from build123d import *

# Parameters (mm, degrees)
SKETCH_2_R          = 1.6
EXTRUDE_1_DEPTH     = 3.8
CUT_EXTRUDE_1_REACH = 22.061
SKETCH_3_R          = 0.925
SKETCH_3_R_2        = 0.7
EXTRUDE_2_DEPTH     = 2


with BuildPart() as part:
    # Эскиз2 → Бобышка-Вытянуть1 (new body)
    with BuildSketch(Plane.XY):
        with BuildLine():
            Line((-14.886464029, 14), (-14.886464029, -14))
            ThreePointArc((-14.886464029, -14), (-10.886464029, -18), (-6.886464029, -14))
            Line((-6.886464029, -14), (-6.886464029, 14))
            ThreePointArc((-6.886464029, 14), (-10.886464029, 18), (-14.886464029, 14))
        make_face()
        with Locations(Location((-10.886464029, -14, 0), (0, 0, 180))):
            Circle(SKETCH_2_R, mode=Mode.SUBTRACT)
        with Locations(Location((-10.886464029, 14, 0), (0, 0, 180))):
            Circle(SKETCH_2_R, mode=Mode.SUBTRACT)
    extrude(amount=EXTRUDE_1_DEPTH)

    # Эскиз3 → Вырез-Вытянуть1 (cut, up to next)
    with BuildSketch(Plane.ZY.offset(14.886464029), mode=Mode.PRIVATE) as cut_extrude_1_sk1:
        with Locations((4, -10)):
            Circle(SKETCH_3_R)
    cut_extrude_1_tool1 = extrude(cut_extrude_1_sk1.sketch, amount=-CUT_EXTRUDE_1_REACH, mode=Mode.PRIVATE) & part.part
    # Эскиз3 → Вырез-Вытянуть1 (cut, up to next)
    with BuildSketch(Plane.ZY.offset(14.886464029), mode=Mode.PRIVATE) as cut_extrude_1_sk2:
        with Locations((4, -7.5)):
            Circle(SKETCH_3_R_2)
    cut_extrude_1_tool2 = extrude(cut_extrude_1_sk2.sketch, amount=-CUT_EXTRUDE_1_REACH, mode=Mode.PRIVATE) & part.part
    # Эскиз3 → Вырез-Вытянуть1 (cut, up to next)
    with BuildSketch(Plane.ZY.offset(14.886464029), mode=Mode.PRIVATE) as cut_extrude_1_sk3:
        with Locations((4, -5)):
            Circle(SKETCH_3_R_2)
    cut_extrude_1_tool3 = extrude(cut_extrude_1_sk3.sketch, amount=-CUT_EXTRUDE_1_REACH, mode=Mode.PRIVATE) & part.part
    # Эскиз3 → Вырез-Вытянуть1 (cut, up to next)
    with BuildSketch(Plane.ZY.offset(14.886464029), mode=Mode.PRIVATE) as cut_extrude_1_sk4:
        with Locations((4, 10)):
            Circle(SKETCH_3_R)
    cut_extrude_1_tool4 = extrude(cut_extrude_1_sk4.sketch, amount=-CUT_EXTRUDE_1_REACH, mode=Mode.PRIVATE) & part.part
    # Эскиз3 → Вырез-Вытянуть1 (cut, up to next)
    with BuildSketch(Plane.ZY.offset(14.886464029), mode=Mode.PRIVATE) as cut_extrude_1_sk5:
        with Locations((4, 7.5)):
            Circle(SKETCH_3_R_2)
    cut_extrude_1_tool5 = extrude(cut_extrude_1_sk5.sketch, amount=-CUT_EXTRUDE_1_REACH, mode=Mode.PRIVATE) & part.part
    # Эскиз3 → Вырез-Вытянуть1 (cut, up to next)
    with BuildSketch(Plane.ZY.offset(14.886464029), mode=Mode.PRIVATE) as cut_extrude_1_sk6:
        with Locations((4, 5)):
            Circle(SKETCH_3_R_2)
    cut_extrude_1_tool6 = extrude(cut_extrude_1_sk6.sketch, amount=-CUT_EXTRUDE_1_REACH, mode=Mode.PRIVATE) & part.part
    # Эскиз3 → Вырез-Вытянуть1 (cut, up to next)
    with BuildSketch(Plane.ZY.offset(14.886464029), mode=Mode.PRIVATE) as cut_extrude_1_sk7:
        with Locations((4, 2.5)):
            Circle(SKETCH_3_R)
    cut_extrude_1_tool7 = extrude(cut_extrude_1_sk7.sketch, amount=-CUT_EXTRUDE_1_REACH, mode=Mode.PRIVATE) & part.part
    # Эскиз3 → Вырез-Вытянуть1 (cut, up to next)
    with BuildSketch(Plane.ZY.offset(14.886464029), mode=Mode.PRIVATE) as cut_extrude_1_sk8:
        with Locations((4, 0)):
            Circle(SKETCH_3_R_2)
    cut_extrude_1_tool8 = extrude(cut_extrude_1_sk8.sketch, amount=-CUT_EXTRUDE_1_REACH, mode=Mode.PRIVATE) & part.part
    # Эскиз3 → Вырез-Вытянуть1 (cut, up to next)
    with BuildSketch(Plane.ZY.offset(14.886464029), mode=Mode.PRIVATE) as cut_extrude_1_sk9:
        with Locations((4, -2.5)):
            Circle(SKETCH_3_R)
    cut_extrude_1_tool9 = extrude(cut_extrude_1_sk9.sketch, amount=-CUT_EXTRUDE_1_REACH, mode=Mode.PRIVATE) & part.part
    add(cut_extrude_1_tool1.solids().sort_by_distance((-14.886464, -10, 4))[0], mode=Mode.SUBTRACT)
    add(cut_extrude_1_tool2.solids().sort_by_distance((-14.886464, -7.5, 4))[0], mode=Mode.SUBTRACT)
    add(cut_extrude_1_tool3.solids().sort_by_distance((-14.886464, -5, 4))[0], mode=Mode.SUBTRACT)
    add(cut_extrude_1_tool4.solids().sort_by_distance((-14.886464, 10, 4))[0], mode=Mode.SUBTRACT)
    add(cut_extrude_1_tool5.solids().sort_by_distance((-14.886464, 7.5, 4))[0], mode=Mode.SUBTRACT)
    add(cut_extrude_1_tool6.solids().sort_by_distance((-14.886464, 5, 4))[0], mode=Mode.SUBTRACT)
    add(cut_extrude_1_tool7.solids().sort_by_distance((-14.886464, 2.5, 4))[0], mode=Mode.SUBTRACT)
    add(cut_extrude_1_tool8.solids().sort_by_distance((-14.886464, 0, 4))[0], mode=Mode.SUBTRACT)
    add(cut_extrude_1_tool9.solids().sort_by_distance((-14.886464, -2.5, 4))[0], mode=Mode.SUBTRACT)

    # Эскиз4 → Бобышка-Вытянуть2 (add)
    with BuildSketch(Plane(origin=(0, 0, 0), x_dir=(-1, 0, 0), z_dir=(0, 0, -1))):
        Polygon((10.886464029, 10.651368439), (13.786464029, 12.325684219), (14.886464029, 12.325684219), (14.886464029, -12.325684219), (13.786464029, -12.325684219), (10.886464029, -10.651368439), (7.986464029, -12.325684219), (6.886464029, -12.325684219), (6.886464029, 12.325684219), (7.986464029, 12.325684219), align=None)
    extrude(amount=EXTRUDE_2_DEPTH)


solid = part.part
Source: CAD feature listing. Evaluate the final solid. Frame: model axes, mm. A direction names the side the tool comes from. Give positions to 0.01 mm unless a question says otherwise; leave off trailing zeros. Write each loop counter-clockwise with the first axis right and the second up, starting at its lowest first coordinate (ties: lowest second). Pieces come first, ordered by that corner, then holes. Notation, with made-up numbers: (0, -13.75) -> (13, -13.75) arc R8 cw to (13, -5.75) -> close; hole circle Ø3 at (15.25, -25). An arc over 180 degrees is marked (long way). Return JSON: item names as keys, results as strings. Group by question number.
1. Section D-D, the plane y = -3. Output: boundary loops of the cut face in (x, z).
2. Access query for faces 1 (the face through (-12.32, 11.48, -0.99)), 2 (the face through (-9.457, -11.477, -0.986)), 3 (the face through (-7.4, 12.326, -1)), 4 (the face through (-10.9, -8.6, 3.8)). Directions: +Z, -Z, +X, -X, +Y, -Y. A direction counts if a zero-diameter tool reaches every point of the face in a straight line with its end or side. Return the directions, or none.
3. Pin query (flat end, axial travel): pin 1 Ø1 at (x, z) = (-13.5, 1.5) entering from +Y; pin 2 Ø0.6 at (x, z) = (-14.5, -1) entering from +Y; pin 3 Ø0.9 at (x, z) = (-14.5, -1.5) entering from -Y; pin 4 Ø2.5 at (x, y) = (-10.89, -14) entering from -Z. Return the tip coordinate at first contact, or that it passes through.
4. Section A-A, the plane z = -0.5. Output: boundary loops of the cut face in (x, y), then the cut area to 4 significant figures.
5. Material intervals for line 1 (Y direction, x = -11, z = 1.85); line 2 (X direction, y = -14, z = 1.75); line 3 (Z direction, x = -10.75, y = -10) (3 decimals), sorted ascending. Write a range as from..to.
6. Section B-B, the plane x = -9.75. Count the separate pieces of the cut face and the enclosed holes in it, then the cut area to 3 significant figures.
7. Section C-C, the plane y = -10. Output: boundary loops of the cut face in (x, z) (3 decimals).
8. Mould query, pull axis X, two halves, no side actions, for faces 5 (the face through (-10.942, -9.982, 3.075)), 6 (the face through (-11, 18, 2)), 7 (the face through (-9.707, -15.081, 1.873)). Classes: +X half, -X half, draft (parallel to the pull), parting line (faces both ways), or undercut.
Determined:
{
 "1": {"outline": "(-14.89, -2) -> (-6.89, -2) -> (-6.89, 3.22) -> (-14.89, 3.22) -> close"},
 "2": {"face 1": "-Z, +Y", "face 2": "-Z, -Y", "face 3": "-Z, +X, -X, +Y", "face 4": "+Z, +X, -X, +Y, -Y"},
 "3": {"pin 1": "stops at y = 17.4", "pin 2": "stops at y = 12.33", "pin 3": "stops at y = -12.33", "pin 4": "passes through"},
 "4": {"outline": "(-14.89, -12.33) -> (-13.79, -12.33) -> (-10.89, -10.65) -> (-7.99, -12.33) -> (-6.89, -12.33) -> (-6.89, 12.33) -> (-7.99, 12.33) -> (-10.89, 10.65) -> (-13.79, 12.33) -> (-14.89, 12.33) -> close", "area": "187.5 mm2"},
 "5": {"line 1": "y = -18..-15.6, -12.4..12.4, 15.6..18", "line 2": "x = -14.89..-12.49, -9.29..-6.89", "line 3": "z = -2..3.075"},
 "6": {"separate pieces": "3", "enclosed holes": "0", "area": "157 mm2"},
 "7": {"outline": "(-14.886, -2) -> (-6.886, -2) -> (-6.886, 3.075) -> (-14.886, 3.075) -> close"},
 "8": {"face 5": "draft", "face 6": "parting line", "face 7": "undercut"}
}
